from build123d import *

# Parameters (mm, degrees)
SKETCH_1_R      = 1.5
SKETCH_1_R_2    = 2
SKETCH_1_R_3    = 1.6
SKETCH_1_R_4    = 1.15
EXTRUDE_1_DEPTH = 5
FILLET_1_R      = 20


with BuildPart() as part:
    # 草图1 → 凸台-拉伸1 (new body)
    with BuildSketch(Plane.XY):
        Polygon((0, 108.239220029), (-76.536686473, 76.536686473), (-108.239220029, 0), (-76.536686473, -76.536686473), (0, -108.239220029), (76.536686473, -76.536686473), (108.239220029, 0), (76.536686473, 76.536686473), align=None)
        with Locations((-46.741505227, -16.11378879)):
            Circle(SKETCH_1_R, mode=Mode.SUBTRACT)
        with Locations((-16.892197502, -88.176392326)):
            Circle(SKETCH_1_R, mode=Mode.SUBTRACT)
        with Locations((74.294712357, -50.405537551)):
            Circle(SKETCH_1_R, mode=Mode.SUBTRACT)
        with Locations((44.445404632, 21.657065985)):
            Circle(SKETCH_1_R, mode=Mode.SUBTRACT)
        with Locations((-35.206875778, -84.996916991)):
            Circle(SKETCH_1_R_2, mode=Mode.SUBTRACT)
        with Locations((84.996916991, -35.206875778)):
            Circle(SKETCH_1_R_2, mode=Mode.SUBTRACT)
        with Locations((35.206875778, 84.996916991)):
            Circle(SKETCH_1_R_2, mode=Mode.SUBTRACT)
        with Locations((-84.996916991, 35.206875778)):
            Circle(SKETCH_1_R_2, mode=Mode.SUBTRACT)
        with Locations((22.421756372, 17.730054744)):
            Circle(SKETCH_1_R_3, mode=Mode.SUBTRACT)
        with Locations((-28.391617917, -3.317534036)):
            Circle(SKETCH_1_R_3, mode=Mode.SUBTRACT)
        with Locations((-49.092265239, 66.256693954)):
            Circle(SKETCH_1_R_3, mode=Mode.SUBTRACT)
        with Locations((-12.137083939, 81.564031248)):
            Circle(SKETCH_1_R_3, mode=Mode.SUBTRACT)
        with Locations((-89.991239438, 8.207996367)):
            Circle(SKETCH_1_R_4, mode=Mode.SUBTRACT)
        with Locations((-77.056925983, 13.56556442)):
            Circle(SKETCH_1_R_4, mode=Mode.SUBTRACT)
        with Locations((-69.939014141, -3.618594885)):
            Circle(SKETCH_1_R_4, mode=Mode.SUBTRACT)
        with Locations((-82.873327596, -8.976162938)):
            Circle(SKETCH_1_R_4, mode=Mode.SUBTRACT)
        with Locations((48.55098737, 78.146027573)):
            Circle(SKETCH_1_R_2, mode=Mode.SUBTRACT)
        with Locations((20.926853617, 89.588318422)):
            Circle(SKETCH_1_R_2, mode=Mode.SUBTRACT)
        with Locations((89.588318422, -20.926853617)):
            Circle(SKETCH_1_R_2, mode=Mode.SUBTRACT)
        with Locations((-48.55098737, -78.146027573)):
            Circle(SKETCH_1_R_2, mode=Mode.SUBTRACT)
        with Locations((-78.146027573, 48.55098737)):
            Circle(SKETCH_1_R_2, mode=Mode.SUBTRACT)
        with Locations((-89.588318422, 20.926853617)):
            Circle(SKETCH_1_R_2, mode=Mode.SUBTRACT)
        with BuildLine():
            Line((-40.596693041, 45.746568332), (-3.64151174, 61.053905626))
            ThreePointArc((-3.64151174, 61.053905626), (22.489747557, 50.229983624), (11.665825554, 24.098724326))
            Line((11.665825554, 24.098724326), (-25.289355746, 8.791387031))
            ThreePointArc((-25.289355746, 8.791387031), (-51.420615044, 19.615309034), (-40.596693041, 45.746568332))
        make_face(mode=Mode.SUBTRACT)
    extrude(amount=EXTRUDE_1_DEPTH)

    # 圆角1
    fillet_1_edges = [part.edges().sort_by_distance(p)[0] for p in [
        (76.536686473, 76.536686473, 2.5),
        (108.239220029, 0, 2.5),
        (76.536686473, -76.536686473, 2.5),
        (0, -108.239220029, 2.5),
        (-76.536686473, -76.536686473, 2.5),
        (-108.239220029, 0, 2.5),
        (-76.536686473, 76.536686473, 2.5),
        (0, 108.239220029, 2.5),
    ]]
    fillet(fillet_1_edges, radius=FILLET_1_R)


solid = part.part
Model file for the job. Use its own axes, mm. Coordinates: 2 decimals unless noted, no trailing zeros. Order: outer loops, then holes, each group sorted by start corner. A loop starts at its lowest first (then second) coordinate and runs counter-clockwise, first axis right, second up. Notation, with made-up numbers: (-40, 79) -> (-5, 79) arc R17 cw to (-5, 107) -> close; hole circle Ø6 at (86.25, 54.25). An arc over 180 degrees is marked (long way). Return JSON: item names as keys, results as strings. Group by question number.
Item 1: Saw through at C-C on y = -55.5. Write the cut outline in (x, z).
Item 2: Pull direction X, two halves, no side cores. Call faces 1 (the flat face through (-22.378, 53.293, 2.465)), 2 (the cylindrical face through (-75.45, -75.29, 2.54)), 3 (the flat face through (38.7, 92.21, 2.46)), 4 (the cylindrical face through (-51.248, 19.211, 2.465)): pulls with the +X half, pulls with the -X half, needs draft (parallel to the pull), parting line crosses it, or undercut.
Item 3: Wall check: line 1 along Y through (x, z) = (-90, 3.15); line 2 along Y through (x, z) = (19.5, 0.8); line 3 along X through (y, z) = (-61, 1.9). Give the ranges that are in metal, low to high. Write a range as [from, to].
Item 4: Saw through at A-A on y = 27. Write the cut outline in (x, z), then the cut area to 3 significant figures.
Item 5: Flat gauge pin, fed straight in: P1, Ø3.5, axis at x = -35.21, y = -85, coming from the -Z side. Where does the tip first touch, or does it go through?
Item 6: Saw through at D-D on y = 72. Write the cut outline in (x, z), then the cut area to 3 significant figures.
Item 7: Saw through at B-B on z = 2.8. State how many separate pieces and enclosed holes the cut face has, then the cut area to 3 significant figures.
Values found:
{
 "1": {"outline": "(-85.25, 0) -> (85.25, 0) -> (85.25, 5) -> (-85.25, 5) -> close"},
 "2": {"face 1": "undercut", "face 2": "pulls with the -X half", "face 3": "pulls with the +X half", "face 4": "undercut"},
 "3": {"line 1": "y = [-44.03, 7.06], [9.36, 18.97], [22.88, 44.03]", "line 2": "y = [-100.16, 29.92], [55.23, 88.19], [90.99, 100.16]", "line 3": "x = [-82.97, 82.97]"},
 "4": {"outline": "(-97.06, 0) -> (-52.94, 0) -> (-52.94, 5) -> (-97.06, 5) -> close; (16.56, 0) -> (97.06, 0) -> (97.06, 5) -> (16.56, 5) -> close", "area": "623 mm2"},
 "5": {"P1": "passes through"},
 "6": {"outline": "(-78.08, 0) -> (78.08, 0) -> (78.08, 5) -> (-78.08, 5) -> close", "area": "781 mm2"},
 "7": {"separate pieces": "1", "enclosed holes": "23", "area": "30,000 mm2"}
}
